The listing builds one solid part. Answer for the finished solid, in the listing's coordinates (mm). Face numbers are marked on the shaded views. A direction names the side the tool comes from. Coordinates: 2 decimals unless noted, no trailing zeros. Order: outer loops, then holes, each group sorted by start corner. A loop starts at its lowest first (then second) coordinate and runs counter-clockwise, first axis right, second up. Notation, with made-up numbers: (-29, 34.5) -> (23, 34.5) arc R20 ccw to (23, 51.5) -> close; hole circle Ø2 at (-9.5, 51). An arc over 180 degrees is marked (long way). Write each question's results on one line, items separated by ' | '. Start each with the question number.
(1) Determine the mould class of the marked faces 4, 5, 6 and 7 for opening direction X: +X half, -X half, draft (parallel to the pull), parting line (faces both ways), or undercut.
(2) The part is cut by section A-A, the plane z = 11.5. Give the vertices of the cut face in (x, y).
(3) The part is cut by section B-B, the plane z = 8.2. Give the vertices of the cut face in (x, y), then the cut area to 3 significant figures.
(4) The part is cut by section D-D, the plane x = 4. Give the vertices of the cut face in (y, z), then the cut area to 4 significant figures.
(5) The part is cut by section C-C, the plane y = -5. Give the vertices of the cut face in (x, z), then the cut area to 3 significant figures.
(6) A tool of negligible diameter and unlimited length cuts with its end or side. For the marked faces 1, 2 and 3, from which of +Z, -Z, +X, -X, +Y, -Y can it reach the whole face along a straight path? Write none if from no direction.
(7) Straight lines are drawn through the part: L1, parallel to X at y = -2, z = 5.25; L2, parallel to Y at x = 12, z = 12.25; L3, parallel to Y at x = 23.1, z = 8.2. For each, find the intervals that lie inside material, in ascending order.
(8) Given pin 1 (10 mm diameter, centred on x = 5, y = 4.5, fed in from +Z); pin 2 (2 mm diameter, centred on x = 6, z = 9, fed in from -Y); pin 3 (3.5 mm diameter, centred on x = 22, z = 5, fed in from -Y), each flat-ended and moving along its own axis, determine where each tip first touches the part or whether it passes through.
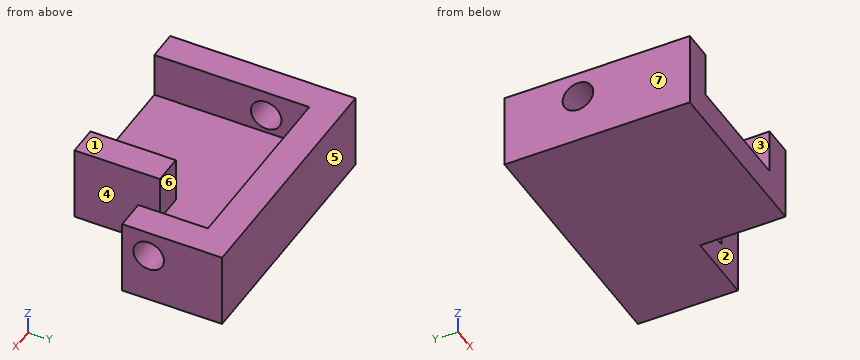
Autodesk Inventor part; units mm, degrees
ref_plane "YZ Plane" through (0, 0, 0) normal (1, 0, 0) x (0, 1, 0)
ref_plane "XZ Plane" through (0, 0, 0) normal (0, 1, 0) x (-1, 0, 0)
ref_plane "XY Plane" through (0, 0, 0) normal (0, 0, 1) x (1, 0, 0)
sketch "Sketch1" plane through (0, 0, 0) normal (0, 0, 1) x (1, 0, 0)
  line L0 (4.1434, -12.66) -> (3.2904, -12.66)
  line L1 (-14.9, 12.8) -> (14.9, 12.8)
  line L2 (14.9, 12.8) -> (14.9, -12.8)
  line L3 (14.9, -12.8) -> (-14.9, -12.8)
  line L4 (-14.9, -12.8) -> (-14.9, 12.8)
  point P0 (0, 0)
  point P1 (0, 12.8)
  point P2 (-14.9, 0)
  dimension "d4" = 29.8
  dimension "d5" = 25.6
extrude "Extrusion1" add sketch "Sketch1" along normal blind 12.5
sketch "Sketch2" plane through (0, 0, 12.5) normal (0, 0, 1) x (1, 0, 0)
  line L0 (-14.9, -12.8) -> (14.9, -12.8)
  line L1 (-9.96, -12.8) -> (9.96, -12.8)
  line L2 (9.96, -12.8) -> (9.96, 7.8)
  line L3 (9.96, 7.8) -> (-9.96, 7.8)
  line L4 (-9.96, 7.8) -> (-9.96, -12.8)
  line L5 (14.9, 12.8) -> (-14.9, 12.8)
  point P0 (0, 0)
  point P1 (0, 7.8)
  dimension "d8" = 19.92
  dimension "d9" = 5
extrude "Extrusion2" cut sketch "Sketch2" against normal blind 7.5
sketch "Sketch3" plane through (0, 0, 12.5) normal (0, 0, 1) x (1, 0, 0)
  line L0 (-0.14, 0.6) -> (-0.84, 1.3)
  line L1 (14.9, -12.8) -> (14.9, 12.8)
  line L2 (14.9, -3.7) -> (26.6432, -3.7)
  line L3 (26.6432, -3.7) -> (26.6432, 12.8)
  line L4 (26.6432, 12.8) -> (14.9, 12.8)
  line L5 (14.9, 12.8) -> (14.9, -3.7)
  line L6 (14.9, 12.8) -> (-14.9, 12.8)
  line L7 (-7.482, 1.9485) -> (17.86, 10.1145)
  line L8 (-7.482, 1.9485) -> (19.1432, 1.9485)
  line L9 (9.96, 7.8) -> (9.96, -12.8)
  line L10 (9.96, 1.3) -> (21.6432, 1.3)
  line L11 (21.6432, 1.3) -> (21.6432, 7.8)
  line L12 (21.6432, 7.8) -> (9.96, 7.8)
  line L13 (9.96, 7.8) -> (9.96, 1.3)
  line L14 (-9.96, 7.8) -> (9.96, 7.8)
  point P0 (0, 0)
  point P1 (15.8016, 1.3)
  point P2 (21.6432, 4.55)
  dimension "d12" = 5
  dimension "d13" = 7.5
  dimension "d14" = 5
extrude "Extrusion3" add sketch "Sketch3" against normal blind 12.5 contours L1 L10 L11 L12 L4 L3 L2 | L1 L12 L11 L10
sketch "Sketch4" plane through (0, 0, 12.5) normal (0, 0, 1) x (1, 0, 0)
  line L0 (21.6432, 7.8) -> (9.96, 7.8)
  line L1 (9.96, 7.8) -> (9.96, 1.3)
  line L2 (9.96, 1.3) -> (21.6432, 1.3)
  line L3 (21.6432, 1.3) -> (21.6432, 7.8)
  point P0 (0, 0)
extrude "Extrusion4" cut sketch "Sketch4" against normal blind 7.5
thicken "Thicken1" operation add thickness 5 both sides no extend neighbours no toward (0, 1, 0) faces at (12.7954, 12.8, 4.1667)
sketch "Sketch5" plane through (0, 0, 12.5) normal (0, 0, 1) x (1, 0, 0)
  line L0 (-9.96, 7.8) -> (21.6432, 7.8)
  line L1 (-9.96, 7.8) -> (21.6432, 7.8)
  line L2 (21.6432, 7.8) -> (21.6432, 12.8)
  line L3 (21.6432, 12.8) -> (-9.96, 12.8)
  line L4 (-9.96, 12.8) -> (-9.96, 7.8)
  line L5 (21.6432, 7.8) -> (21.6432, 1.3)
  point P0 (0, 0)
  dimension "d21" = 5
extrude "Extrusion5" cut sketch "Sketch5" against normal blind 7.5
sketch "Sketch6" plane through (-14.9, -12.8, 0) normal (-1, 0, 0) x (0, 0, 1)
  circle A0 centre (8.2, 18.4735) radius 2.525
  line L0 (10, 14.7485) -> (6.4, 14.7485)
  line L1 (6.6, 15.3) -> (9.8, 15.3)
  point P0 (0, 12.8)
  point P1 (8.2, 14.7485)
  point P2 (8.2, 15.9485)
  dimension "d24" = 5.05
  dimension "d25" = 1.2
extrude "Extrusion6" cut sketch "Sketch6" against normal through all
sketch "Sketch7" plane through (0, 0, 12.5) normal (0, 0, 1) x (1, 0, 0)
  line L0 (14.9, -3.7) -> (26.6432, -3.7)
  line L1 (26.6432, -3.7) -> (26.6432, 17.8)
  line L2 (14.9, -3.7) -> (26.6432, -3.7)
  line L3 (26.6432, -3.7) -> (26.6432, 1.3)
  line L4 (26.6432, 1.3) -> (14.9, 1.3)
  line L5 (14.9, 1.3) -> (14.9, -3.7)
  point P0 (0, 0)
  dimension "d28" = 5
extrude "Extrusion7" cut sketch "Sketch7" against normal through all
properties part number "SS-5FL111-3T_Housing_01"
Established:
1) face 4: +X half | face 5: draft | face 6: undercut | face 7: -X half
2) outline: (-14.9, -12.8) -> (-9.96, -12.8) -> (-9.96, 12.8) -> (21.64, 12.8) -> (21.64, 1.3) -> (26.64, 1.3) -> (26.64, 17.8) -> (-14.9, 17.8) -> close; (9.96, -12.8) -> (14.9, -12.8) -> (14.9, 1.3) -> (9.96, 1.3) -> close
3) outline: (-14.9, -12.8) -> (-9.96, -12.8) -> (-9.96, 3.15) -> (-14.9, 3.15) -> close; (-14.9, 8.2) -> (-9.96, 8.2) -> (-9.96, 12.8) -> (21.64, 12.8) -> (21.64, 8.2) -> (26.64, 8.2) -> (26.64, 17.8) -> (-14.9, 17.8) -> close; (9.96, -12.8) -> (14.9, -12.8) -> (14.9, 1.3) -> (9.96, 1.3) -> close; (21.64, 1.3) -> (26.64, 1.3) -> (26.64, 3.15) -> (21.64, 3.15) -> close | area: 411 mm^2
4) outline: (-12.8, 0) -> (17.8, 0) -> (17.8, 12.5) -> (12.8, 12.5) -> (12.8, 5) -> (-12.8, 5) -> close | area: 190.5 mm^2
5) outline: (-14.9, 0) -> (14.9, 0) -> (14.9, 12.5) -> (9.96, 12.5) -> (9.96, 5) -> (-9.96, 5) -> (-9.96, 12.5) -> (-14.9, 12.5) -> close | area: 223 mm^2
6) face 1: +Z, +X, -X, +Y, -Y | face 2: +Z, -Z, +X, -Y | face 3: +Z, -Y
7) L1: x = -14.9 to -9.96, 9.96 to 14.9 | L2: y = -12.8 to 1.3, 12.8 to 17.8 | L3: y = 1.3 to 3.15, 8.2 to 17.8
8) pin 1: stops at z = 5 | pin 2: stops at y = 12.8 | pin 3: stops at y = 1.3
